```python
from build123d import *

# Parameters (mm, degrees)
BOSS_EXTRUDE1_DEPTH      = 12.5
BOSS_EXTRUDE1_DEPTH_BACK = 12.5
SKETCH3_R                = 4
SKETCH3_R_2              = 2.1
CHAMFER1_SIZE            = 0.19
CHAMFER2_SIZE            = 0.285


with BuildPart() as part:
    # Sketch3 → Boss-Extrude1 (new, two sides: drawn at the far end of the back side and taken through both)
    with BuildSketch(Plane.XY.offset(-BOSS_EXTRUDE1_DEPTH_BACK)):
        Circle(SKETCH3_R)
        Circle(SKETCH3_R_2, mode=Mode.SUBTRACT)
    extrude(amount=BOSS_EXTRUDE1_DEPTH + BOSS_EXTRUDE1_DEPTH_BACK)

    # Chamfer1
    chamfer1_edges = [part.edges().sort_by_distance(p)[0] for p in [
        (-4, 0, -12.5),
        (-4, 0, 12.5),
    ]]
    chamfer(chamfer1_edges, length=CHAMFER1_SIZE)

    # Chamfer2
    chamfer2_edges = [part.edges().sort_by_distance(p)[0] for p in [
        (-2.1, 0, -12.5),
        (-2.1, 0, 12.5),
    ]]
    chamfer(chamfer2_edges, length=CHAMFER2_SIZE)


solid = part.part
```
Check sheet for the modelled part. Datum: model origin and axes. Units: mm. Coordinates: 2 decimals unless noted, no trailing zeros. Loops run counter-clockwise (first coordinate to the right, second up) from the corner with the lowest first, then second, coordinate; pieces in that order, holes last. Notation, with made-up numbers: M -6.5,18 L 2.5,18 A13 cw 2.5,41 Z; hole C 68.5,-38 d4. An arc over 180 degrees is marked long. Answer as a JSON object with one key per item and string values.
1. Scan lines: L1, parallel to Y at x = 0, z = 1; L2, parallel to X at y = -0.5, z = -5.25; L3, parallel to X at y = -1.5, z = 10.75. Record each from-to range of solid material in increasing order. Write a range as from..to.
Outcome:
{"L1": "-4..-2.1, 2.1..4", "L2": "-3.97..-2.04, 2.04..3.97", "L3": "-3.71..-1.47, 1.47..3.71"}
2. Release check for a two-part mould opening along X. For faces 1 (the flat face through (-2, -2, 12.5)), 2 (the cylindrical face through (-0.867, -3.905, -0.172)), 3 (the cylindrical face through (2.003, 0.631, -0.171)) record: pulls with the +X half, pulls with the -X half, needs draft (parallel to the pull), parting line crosses it, or undercut.
Outcome:
{"face 1": "needs draft", "face 2": "parting line crosses it", "face 3": "undercut"}
3. Sectioned sample at A-A on y = 0. Record the cut outline in (x, z) (3 decimals), and give its area (3 significant figures).
Outcome:
{"outline": "M -4,-12.31 L -3.81,-12.5 L -2.385,-12.5 L -2.1,-12.215 L -2.1,12.215 L -2.385,12.5 L -3.81,12.5 L -4,12.31 Z; M 2.1,-12.215 L 2.385,-12.5 L 3.81,-12.5 L 4,-12.31 L 4,12.31 L 3.81,12.5 L 2.385,12.5 L 2.1,12.215 Z", "area": "94.8 mm²"}
4. Sectioned sample at C-C on z = 10. Record the cut outline in (x, y), and give its area (3 significant figures).
Outcome:
{"outline": "C 0,0 d8; hole C 0,0 d4.2", "area": "36.4 mm²"}
5. Depth check by flat-ended pin: P1, Ø1.5, axis at x = -1, z = 1.5, coming from the +Y side; P2, Ø1, axis at y = -1, z = 6, coming from the -X side; P3, Ø3, axis at y = -3, z = 4.5, coming from the +X side. Enter the tip coordinate at first touch or a pass-through.
Outcome:
{"P1": "y = 3.99", "P2": "x = -3.97", "P3": "x = 3.71"}
